Geometry: final body of the model. Coordinates: model frame, mm. A direction names the side the tool comes from. Coordinates: 2 decimals unless noted, no trailing zeros. Write each loop counter-clockwise with the first axis right and the second up, starting at its lowest first coordinate (ties: lowest second). Pieces come first, ordered by that corner, then holes.
from build123d import *

# Parameters (mm, degrees)
SKETCH_1_R               = 118
SKETCH_1_R_2             = 113
EXTRUDE_1_DEPTH          = 11
EXTRUDE_START            = -3
SKETCH_2_W               = 15
SKETCH_2_H               = 98.117087724
EXTRUDE_2_DEPTH          = 4
PATTERN_CIRCULAR_1_COUNT = 6
EXTRUDE_3_DEPTH          = 3
EXTRUDE_3_DEPTH_BACK     = 3
SKETCH_3_R               = 22
SKETCH_3_R_2             = 7


with BuildPart() as part:
    # 草图1 → 拉伸-薄壁1 (new body)
    with BuildSketch(Plane.XY):
        Circle(SKETCH_1_R)
        Circle(SKETCH_1_R_2, mode=Mode.SUBTRACT)
    extrude(amount=EXTRUDE_1_DEPTH)

    # 草图2 → 拉伸-薄壁2 (add)
    with BuildSketch(Plane.XY.offset(11).offset(EXTRUDE_START)):
        with Locations((0, 63.941456138)):
            Rectangle(SKETCH_2_W, SKETCH_2_H)
    extrude_2 = extrude(amount=EXTRUDE_2_DEPTH)

    # 阵列(圆周)1: 拉伸-薄壁2 ×6 about axis
    pattern_circular_1_axis = Axis((0, 0, 0), (0, 0, 1))
    for i in range(1, PATTERN_CIRCULAR_1_COUNT):
        add(extrude_2.rotate(pattern_circular_1_axis, i * 360 / PATTERN_CIRCULAR_1_COUNT))

    # 草图3 → 拉伸-薄壁3 (add, two sides: drawn at the far end of the back side and taken through both)
    with BuildSketch(Plane.XY.offset(11).offset(-EXTRUDE_3_DEPTH_BACK)):
        Circle(SKETCH_3_R)
        Circle(SKETCH_3_R_2, mode=Mode.SUBTRACT)
    extrude(amount=EXTRUDE_3_DEPTH + EXTRUDE_3_DEPTH_BACK)


solid = part.part
Item 1: Pull-direction query (X, two-part tool) for faces 4 (the flat face through (-8, 1, 8)), 5 (the flat face through (97.913, -56.409, 11.493)), 6 (the flat face through (-58, -34, 12)), 7 (the flat face through (-97.81, -56.59, 11.49)); classes: released by +X, released by -X, zero draft, split by the parting line, or undercut.
Derived:
face 4: undercut
face 5: released by +X
face 6: zero draft
face 7: released by -X
Item 2: Section D-D, the plane x = 0. Output: boundary loops of the cut face in (y, z).
Derived:
outline: (-118, 0) - (-113, 0) - (-113, 8) - (-7, 8) - (-7, 14) - (-22, 14) - (-22, 12) - (-113, 12) - (-113, 11) - (-118, 11) - close; (7, 8) - (113, 8) - (113, 0) - (118, 0) - (118, 11) - (113, 11) - (113, 12) - (22, 12) - (22, 14) - (7, 14) - close
Item 3: Material intervals for probe 1 along Y at (x, z) = (-84, 9.75); probe 2 along Y at (x, z) = (-24.5, 9.25); probe 3 along Y at (x, z) = (0, 2.25), sorted ascending.
Derived:
probe 1: y = -82.87 to -75.58, -57.16 to -39.84, 39.84 to 57.16, 75.58 to 82.87
probe 2: y = -115.43 to -110.31, -22.81 to -5.48, 5.48 to 22.81, 110.31 to 115.43
probe 3: y = -118 to -113, 113 to 118
Item 4: Set-up query: faces 1 (the flat face through (61.076, 26.602, 9.972)), 2 (the flat face through (96, -61, 0)), 3 (the flat face through (97.81, 56.59, 11.49)). Return all of +Z, -Z, +X, -X, +Y, -Y with unobstructed straight access to the full face (end or side cutting, diameter ignored); none if empty.
Derived:
face 1: +Z, -Z
face 2: -Z, +X, -X, +Y, -Y
face 3: +Z, +X, +Y
Item 5: Section A-A, the plane y = 0. Output: boundary loops of the cut face in (x, z).
Derived:
outline: (-118, 0) - (-113, 0) - (-113, 11) - (-118, 11) - close; (-22, 8) - (-7, 8) - (-7, 14) - (-22, 14) - close; (7, 8) - (22, 8) - (22, 14) - (7, 14) - close; (113, 0) - (118, 0) - (118, 11) - (113, 11) - close
Item 6: Section C-C, the plane y = 38. Output: boundary loops of the cut face in (x, z).
Derived:
outline: (-111.71, 0) - (-106.42, 0) - (-106.42, 11) - (-111.71, 11) - close; (-80.82, 8) - (-50.82, 8) - (-50.82, 12) - (-80.82, 12) - close; (-7.5, 8) - (7.5, 8) - (7.5, 12) - (-7.5, 12) - close; (50.82, 8) - (80.82, 8) - (80.82, 12) - (50.82, 12) - close; (106.42, 0) - (111.71, 0) - (111.71, 11) - (106.42, 11) - close
Item 7: Pin query (flat end, axial travel): pin 1 (0.8 mm diameter, centred on x = 0.5, z = 11.5, fed in from -Y); pin 2 (2 mm diameter, centred on y = -78.5, z = 9.5, fed in from -X); pin 3 (4.5 mm diameter, centred on y = 59.5, z = 10, fed in from -X). Return the tip coordinate at first contact, or that it passes through.
Derived:
pin 1: stops at y = -113
pin 2: stops at x = -88.98
pin 3: stops at x = -103.18
Item 8: Section B-B, the plane x = -64. Output: boundary loops of the cut face in (y, z).
Derived:
outline: (-99.14, 0) - (-93.13, 0) - (-93.13, 11) - (-99.14, 11) - close; (-45.61, 8) - (-28.29, 8) - (-28.29, 12) - (-45.61, 12) - close; (28.29, 8) - (45.61, 8) - (45.61, 12) - (28.29, 12) - close; (93.13, 0) - (99.14, 0) - (99.14, 11) - (93.13, 11) - close
